Source: three-view drawing plus pictorial views. Frame: mm from the lowest corner of the part. A direction names the side the tool comes from. Coordinates: 2 decimals unless noted, no trailing zeros. Write each loop counter-clockwise with the first axis right and the second up, starting at its lowest first coordinate (ties: lowest second). Pieces come first, ordered by that corner, then holes. Notation, with made-up numbers: (60, 48) -> (102, 48) arc R12 cw to (102, 57) -> close; hole circle Ø1 at (-20.5, 71.25). An arc over 180 degrees is marked (long way). One line per item, written item: value.
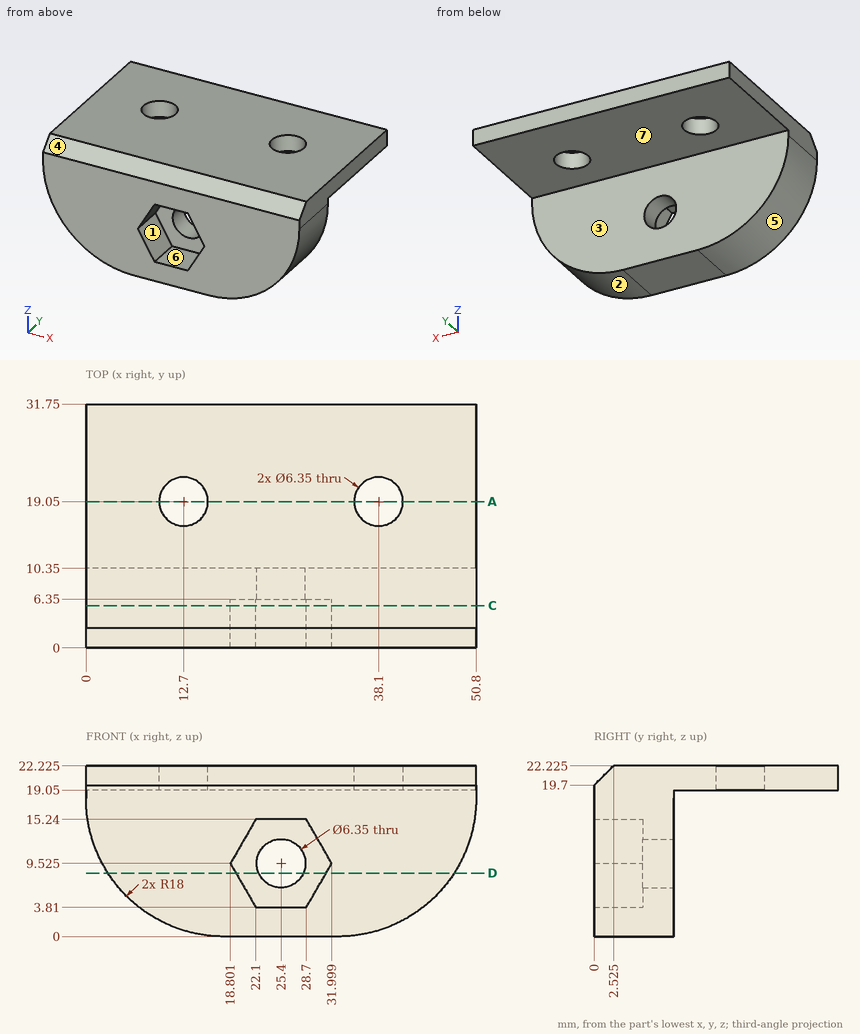
(1) Reachability of the marked faces 5, 6 and 7 from +Z, -Z, +X, -X, +Y, -Y: full face, straight path, thin tool, end or side. Return the list, or none.
Responses:
face 5: -Z, -X, +Y, -Y
face 6: -Y
face 7: -Z, +X, -X, +Y
(2) Pull-direction query (Z, two-part tool) for the marked faces 1, 2, 3 and 4; classes: released by +Z, released by -Z, zero draft, split by the parting line, or undercut.
Responses:
face 1: undercut
face 2: released by -Z
face 3: zero draft
face 4: released by +Z
(3) Line query: line 1 (Y direction, x = 33, z = 14.5); line 2 (Y direction, x = 22, z = 12.75); line 3 (X direction, y = 6.5, z = 11). Output: solid intervals per line, ascending. Write a range as [from, to].
Responses:
line 1: y = [0, 10.35]
line 2: y = [6.35, 10.35]
line 3: x = [1.42, 22.59], [28.21, 49.38]
(4) Section D-D (z = 8.25). Return the cut outline in (x, y), then the cut area to 3 significant figures.
Responses:
outline: (2.87, 0) -> (19.54, 0) -> (19.54, 6.35) -> (22.49, 6.35) -> (22.49, 10.35) -> (2.87, 10.35) -> close; (28.31, 6.35) -> (31.26, 6.35) -> (31.26, 0) -> (47.93, 0) -> (47.93, 10.35) -> (28.31, 10.35) -> close
area: 369 mm2
(5) First-contact query: pin 1 (7.5 mm diameter, centred on x = 12.7, y = 19.05, fed in from -Z); pin 2 (5.5 mm diameter, centred on x = 22.5, z = 10, fed in from -Y); pin 3 (9.5 mm diameter, centred on x = 23.5, z = 12.5, fed in from +Y). Flat tips, straight axial feed; report the tip coordinate or a pass-through.
Responses:
pin 1: stops at z = 19.05
pin 2: stops at y = 6.35
pin 3: stops at y = 10.35
(6) Section C-C (y = 5.5). Return the cut outline in (x, z) (1 decimal).
Responses:
outline: (0, 18) arc R18 ccw to (18, 0) -> (32.8, 0) arc R18 ccw to (50.8, 18) -> (50.8, 22.2) -> (0, 22.2) -> close; hole (18.8, 9.5) -> (22.1, 3.8) -> (28.7, 3.8) -> (32, 9.5) -> (28.7, 15.2) -> (22.1, 15.2) -> close
(7) Section A-A (y = 19.05). State how many separate pieces and enclosed holes the cut face has, then the cut area to 3 significant figures.
Responses:
separate pieces: 3
enclosed holes: 0
area: 121 mm2
